The model under review builds one solid part; all positions refer to its coordinate system, in mm. A direction names the side the tool comes from. Coordinates: 2 decimals unless noted, no trailing zeros. Order: outer loops, then holes, each group sorted by start corner. A loop starts at its lowest first (then second) coordinate and runs counter-clockwise, first axis right, second up.
from build123d import *

# Parameters (mm, degrees)
F1_DEPTH = 23
F2_W     = 33
F2_H     = 3.5
F3_DEPTH = 35
F5_DEPTH = 33
F6_R     = 2.5
F7_R     = 1.7


with BuildPart() as f1:
    # F0 (on Front) → F1 (new body)
    with BuildSketch(Plane.XZ):
        Polygon((-53.5, 32.94), (-53.5, 29.44), (-3.5, 29.44), (-3.5, 3.5), (-53.5, 3.5), (-53.5, 0), (0, 0), (0, 32.94), align=None)
    extrude(amount=F1_DEPTH)

    # F2 (on face) → F3 (join)
    with BuildSketch(Plane(origin=(0, 0, 0), x_dir=(1, 0, 0), z_dir=(0, 0, -1))):
        with Locations((-37, 1.75)):
            Rectangle(F2_W, F2_H)
    extrude(amount=F3_DEPTH)

    # F4 (on face) → F5 (join, through all)
    with BuildSketch(Plane.YZ.offset(-20.5)):
        Polygon((-33.6520012122, -29.6833886639), (-3.5, -35), (-3.5, -31.4460068584), (-33.0442325904, -26.2365615284), align=None)
    extrude(amount=-F5_DEPTH)

    # F6
    f6_edges = [f1.edges().sort_by_distance(p)[0] for p in [
        (-53.5, -11.5, 32.94),
        (0, -11.5, 32.94),
        (0, -11.5, 0),
    ]]
    fillet(f6_edges, radius=F6_R)

    # F7
    f7_edges = [f1.edges().sort_by_distance(p)[0] for p in [
        (-37, -33.652001, -29.683389),
        (-37, -33.044233, -26.236562),
        (-20.5, -18.272116, -28.841284),
        (-53.5, -18.272116, -28.841284),
        (-20.5, -3.5, -15.723003),
        (-37, -3.5, 0),
        (-53.5, -13.25, 0),
        (-53.5, -3.5, -15.723003),
        (-20.5, -1.75, 0),
    ]]
    fillet(f7_edges, radius=F7_R)


solid = f1.part
(1) The part is to be moulded in two halves that separate along Z. For faces 1 (the face through (-33, 0, -1)), 2 (the face through (-37, -3.5, -16)), 3 (the face through (-19.989, -0.913, -0.485)), say which applies: +Z half, -Z half, draft (parallel to the pull), parting line (faces both ways), or undercut.
(2) Consider section C-C (z = 10). Give the boundary of the cut face in (x, y), then the cut area to 3 significant figures.
(3) Consider section B-B (z = -21). Give the boundary of the cut face in (x, y), then the cut area to 3 significant figures.
(4) Insertion check: pin 1 Ø10 at (y, z) = (-12, -24) entering from +X (3 decimals); pin 2 Ø3 at (x, y) = (-21.5, -23.5) entering from -Z; pin 3 Ø2 at (x, y) = (-6, -23.5) entering from -Z; pin 4 Ø1.5 at (y, z) = (-5.5, -0.5) entering from +X. Each pin has a flat end and moves straight along its axis. Give the tip position at first contact, or say it passes through.
(5) Tool access review of faces 4 (the face through (-20.5, -12, -32)), 5 (the face through (-29, -11, 29.44)), 6 (the face through (-53.015, -2.989, -17.808)), 7 (the face through (-52.989, -14.225, 0.485)): name each direction out of +Z, -Z, +X, -X, +Y, -Y from which nothing blocks a thin tool from reaching the whole face with its end or side.
(6) Consider section A-A (x = -8). Give the boundary of the cut face in (y, z).
(7) Wall thickness on line 1 (Z direction, x = -19.5, y = -14.5); line 2 (Z direction, x = -26.5, y = -8.5); line 3 (Z direction, x = -39, y = -2): over which ranges is each line inside the solid? List them lowest first.
Findings:
1. face 1: draft
1. face 2: undercut
1. face 3: -Z half
2. outline: (-3.5, -23) - (0, -23) - (0, 0) - (-3.5, 0) - close
2. area: 80.5 mm2
3. outline: (-53.5, -1.8) arc R1.7 ccw to (-51.8, -3.5) - (-22.2, -3.5) arc R1.7 ccw to (-20.5, -1.8) - (-20.5, 0) - (-53.5, 0) - close
3. area: 114 mm2
4. pin 1: passes through
4. pin 2: stops at z = -31.74
4. pin 3: stops at z = 0
4. pin 4: stops at x = -1.41
5. face 4: -Z, +X, +Y, -Y
5. face 5: -X, +Y, -Y
5. face 6: -X
5. face 7: -X, -Y
6. outline: (-23, 0) - (0, 0) - (0, 3.5) - (-23, 3.5) - close; (-23, 29.44) - (0, 29.44) - (0, 32.94) - (-23, 32.94) - close
7. line 1: z = 0 to 3.5, 29.44 to 32.94
7. line 2: z = -34.12 to -30.56, 0 to 3.5, 29.44 to 32.94
7. line 3: z = -35 to 3.5, 29.44 to 32.94
